from build123d import *

# Parameters (mm, degrees)
SKETCH1_W           = 30
SKETCH1_H           = 15
SKETCH1_R           = 1
SKETCH1_R_2         = 2.38125
BOSS_EXTRUDE1_DEPTH = 5
SKETCH2_R           = 3
CUT_EXTRUDE1_DEPTH  = 2.5


with BuildPart() as part:
    # Sketch1 → Boss-Extrude1 (new body)
    with BuildSketch(Plane.XY):
        Rectangle(SKETCH1_W, SKETCH1_H)
        Circle(SKETCH1_R, mode=Mode.SUBTRACT)
        with Locations((10, 0)):
            Circle(SKETCH1_R_2, mode=Mode.SUBTRACT)
        with Locations((-10, 0)):
            Circle(SKETCH1_R_2, mode=Mode.SUBTRACT)
    extrude(amount=BOSS_EXTRUDE1_DEPTH)

    # Sketch2 → Cut-Extrude1 (cut)
    with BuildSketch(Plane.XY.offset(5)):
        Circle(SKETCH2_R)
    extrude(amount=-CUT_EXTRUDE1_DEPTH, mode=Mode.SUBTRACT)


solid = part.part
Work out the finished part from the listing and answer in its coordinate system (mm). A direction names the side the tool comes from. Give positions to 0.01 mm unless a question says otherwise; leave off trailing zeros. Order: outer loops, then holes, each group sorted by start corner. A loop starts at its lowest first (then second) coordinate and runs counter-clockwise, first axis right, second up. Notation, with made-up numbers: M 79.25,71.5 L 91.25,71.5 A26 cw 91.25,102.5 Z; hole C 54,83.25 d8. An arc over 180 degrees is marked long. Return JSON: item names as keys, results as strings.
Q1. The mould has two halves that part along X. Classify faces 3 (the face through (7.62, 0.1, 2.46)), 4 (the face through (0, -7.5, 2)), 5 (the face through (-15, 0, 2)), 6 (the face through (-3, 0, 4)): pulls with the +X half, pulls with the -X half, needs draft (parallel to the pull), parting line crosses it, or undercut.
Answer below:
{"face 3": "undercut", "face 4": "needs draft", "face 5": "pulls with the -X half", "face 6": "undercut"}
Q2. Find section A-A, the plane x = -10. Write down the section's boundary in (y, z), and give its area (3 significant figures).
Answer below:
{"outline": "M -7.5,0 L -2.38,0 L -2.38,5 L -7.5,5 Z; M 2.38,0 L 7.5,0 L 7.5,5 L 2.38,5 Z", "area": "51.2 mm^2"}
Q3. Find section D-D, the plane x = 0. Write down the section's boundary in (y, z), and give its area (3 significant figures).
Answer below:
{"outline": "M -7.5,0 L -1,0 L -1,2.5 L -3,2.5 L -3,5 L -7.5,5 Z; M 1,0 L 7.5,0 L 7.5,5 L 3,5 L 3,2.5 L 1,2.5 Z", "area": "55.0 mm^2"}
Q4. This flat-tipped pin is pushed along its axis until it touches: pin 1 (1.8 mm diameter, centred on x = 0, y = 0, fed in from +Z). Where does it stop, or does it pass through?
Answer below:
{"pin 1": "passes through"}
Q5. Which of the six approach directions +Z, -Z, +X, -X, +Y, -Y give full straight-line access (tool end or side, diameter ignored) to faces 1 (the face through (0, 2, 0)), 2 (the face through (-1, 1, 2.5))?
Answer below:
{"face 1": "-Z, +X, -X, +Y, -Y", "face 2": "+Z"}
Q6. Find section B-B, the plane z = 0.8. Write down the section's boundary in (x, y), and give its area (3 significant figures).
Answer below:
{"outline": "M -15,-7.5 L 15,-7.5 L 15,7.5 L -15,7.5 Z; hole C -10,0 d4.76; hole C 0,0 d2; hole C 10,0 d4.76", "area": "411 mm^2"}
Q7. Find the intervals of material crossed by line 1 along Y through (x, z) = (0, 1.1); line 2 along X through (y, z) = (-2, 2.8); line 3 along Y through (x, z) = (0, 3.75), in increasing order. Write a range as [from, to].
Answer below:
{"line 1": "y = [-7.5, -1], [1, 7.5]", "line 2": "x = [-15, -11.29], [-8.71, -2.24], [2.24, 8.71], [11.29, 15]", "line 3": "y = [-7.5, -3], [3, 7.5]"}
Q8. Find section C-C, the plane y = 0. Write down the section's boundary in (x, z), and give its area (3 significant figures).
Answer below:
{"outline": "M -15,0 L -12.38,0 L -12.38,5 L -15,5 Z; M -7.62,0 L -1,0 L -1,2.5 L -3,2.5 L -3,5 L -7.62,5 Z; M 1,0 L 7.62,0 L 7.62,5 L 3,5 L 3,2.5 L 1,2.5 Z; M 12.38,0 L 15,0 L 15,5 L 12.38,5 Z", "area": "82.4 mm^2"}
